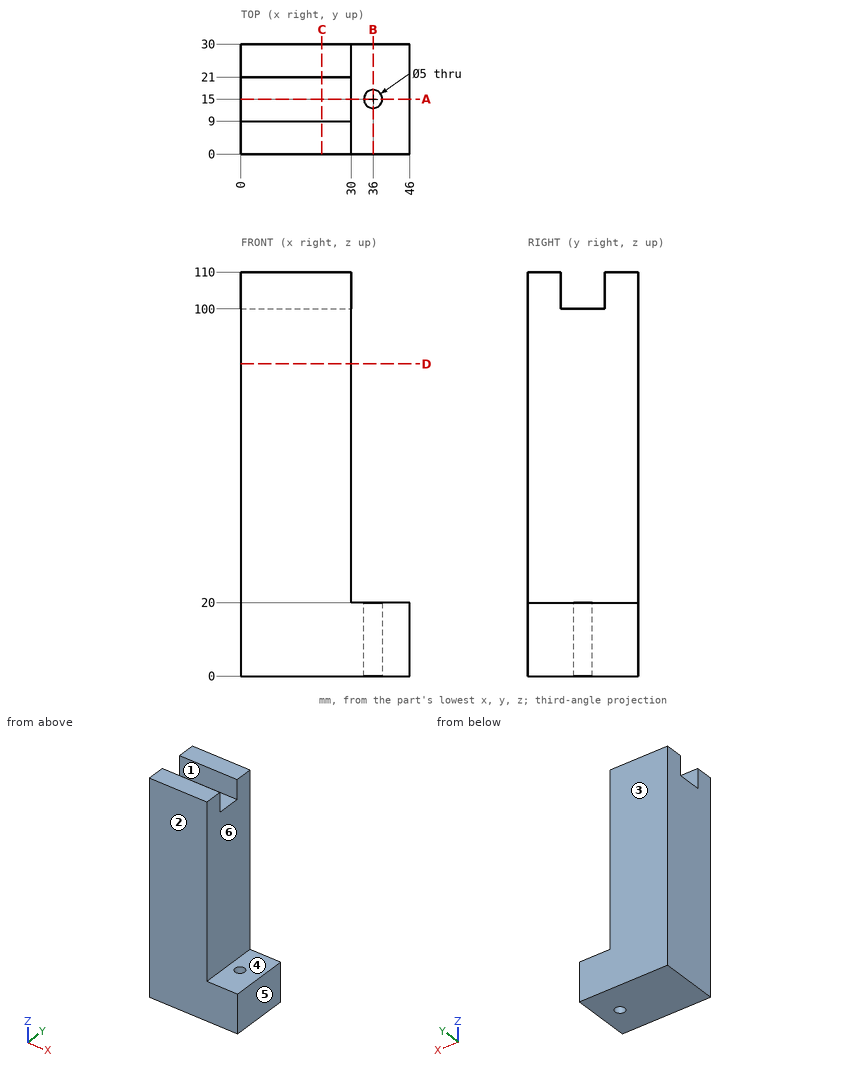
For this review, use the dimensioned drawing (mm, ordinates from the lowest corner) and the shaded views. A direction names the side the tool comes from. Coordinates: 2 decimals unless noted, no trailing zeros. Loops run counter-clockwise (first coordinate to the right, second up) from the corner with the lowest first, then second, coordinate; pieces in that order, holes last. Notation, with made-up numbers: (-16.75, 6) -> (5.25, 6) arc R8 cw to (5.25, 13) -> close; hole circle Ø1 at (37, -9.75). An arc over 180 degrees is marked (long way). Use a Markdown table: item, result. Add a question column.
Item 1: Wall thickness on L1, parallel to X at y = 22.5, z = 23; L2, parallel to Y at x = 36, z = 7; L3, parallel to Z at x = 23, y = 16.75: over which ranges is each line inside the solid? List them lowest first. Write a range as from..to.
Item 2: We need section B-B, the plane x = 36. Write out the cut boundary in (y, z), and give its area (3 significant figures).
Item 3: We need section A-A, the plane y = 15. Write out the cut boundary in (x, z), and give its area (3 significant figures).
Item 4: Clearance check with flat-ended pins moving along their axes: P1, Ø8, axis at x = 12, z = 106.5, coming from the -Y side; P2, Ø3.5, axis at x = 14, y = 14, coming from the +Z side; P3, Ø3, axis at x = 34.5, y = 14.5, coming from the +Z side; P4, Ø10, axis at y = 18.5, z = 82, coming from the +X side. State where each tip first meets the part, or that it passes through.
Item 5: Machinability: for the marked faces 5 and 6, which of the approach directions +Z, -Z, +X, -X, +Y, -Y give a long, thin tool a straight path to every point of the face, cutting with its end or side? Answer none if there is none.
Item 6: We need section C-C, the plane x = 22. Write out the cut boundary in (y, z), and give its area (3 significant figures).
Item 7: The part is to be moulded in two halves that separate along Y. For the marked faces 1, 2, 3 and 4, say which applies: +Y half, -Y half, draft (parallel to the pull), parting line (faces both ways), or undercut.
Item 8: We need section D-D, the plane z = 85. Write out the cut boundary in (x, y), and give its area (3 significant figures).
Numbers:
| question | item | result |
|---|---|---|
| 1 | L1 | x = 0..30 |
| 1 | L2 | y = 0..12.5, 17.5..30 |
| 1 | L3 | z = 0..100 |
| 2 | outline | (0, 0) -> (12.5, 0) -> (12.5, 20) -> (0, 20) -> close; (17.5, 0) -> (30, 0) -> (30, 20) -> (17.5, 20) -> close |
| 2 | area | 500 mm^2 |
| 3 | outline | (0, 0) -> (33.5, 0) -> (33.5, 20) -> (30, 20) -> (30, 100) -> (0, 100) -> close; (38.5, 0) -> (46, 0) -> (46, 20) -> (38.5, 20) -> close |
| 3 | area | 3,220 mm^2 |
| 4 | P1 | stops at y = 0 |
| 4 | P2 | stops at z = 100 |
| 4 | P3 | stops at z = 20 |
| 4 | P4 | stops at x = 30 |
| 5 | face 5 | +Z, -Z, +X, +Y, -Y |
| 5 | face 6 | +Z, +X, +Y, -Y |
| 6 | outline | (0, 0) -> (30, 0) -> (30, 110) -> (21, 110) -> (21, 100) -> (9, 100) -> (9, 110) -> (0, 110) -> close |
| 6 | area | 3,180 mm^2 |
| 7 | face 1 | undercut |
| 7 | face 2 | -Y half |
| 7 | face 3 | +Y half |
| 7 | face 4 | draft |
| 8 | outline | (0, 0) -> (30, 0) -> (30, 30) -> (0, 30) -> close |
| 8 | area | 900 mm^2 |
